Could you check a few things on this model? Use its own coordinates, in mm. Face numbers are marked on the shaded views. Coordinates: 2 decimals unless noted, no trailing zeros. Loops run counter-clockwise (first coordinate to the right, second up) from the corner with the lowest first, then second, coordinate; pieces in that order, holes last.
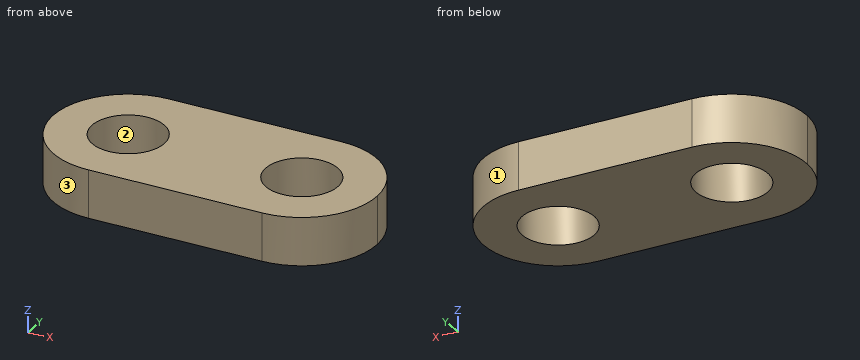
Autodesk Inventor part; units mm, degrees
ref_plane "YZ Plane" through (0, 0, 0) normal (1, 0, 0) x (0, 1, 0)
ref_plane "XZ Plane" through (0, 0, 0) normal (0, 1, 0) x (-1, 0, 0)
ref_plane "XY Plane" through (0, 0, 0) normal (0, 0, 1) x (1, 0, 0)
sketch "Sketch2" plane through (0, 0, 0) normal (0, 1, 0) x (-1, 0, 0)
  line L0 (0, -4.5) -> (-30.1, -4.5)
  line L1 (-30.1, -4.5) -> (-30.1, 0)
  line L2 (-30.1, 0) -> (0, 0)
  line L3 (0, 0) -> (0, -4.5)
  line L4 (-7, -4.5) -> (-7, 0) construction
  line L5 (-23.1, 0) -> (-23.1, -4.5) construction
  point P0 (-7, -2.25)
  point P1 (-23.1, -2.25)
  dimension "d7" = 16.1
  dimension "d8" = 4.5
  dimension "d9" = 7
  dimension "d11" = 7
extrude "Extrusion1" add sketch "Sketch2" along normal blind 14
sketch "Sketch3" plane through (0, 0, 0) normal (0, 0, 1) x (1, 0, 0)
  line L0 (30.1, 0) -> (30.1, 14)
  line L1 (0, 0) -> (0, 14)
  point P0 (7, 7)
  point P1 (23.1, 7)
  point P2 (30.1, 7)
  point P3 (7, 0)
  point P4 (23.1, 0)
hole "Hole1" at (7, 7, 0) at (23.1, 7, 0) direction (0, 0, -1) diameter 6.756 end through all
fillet "Fillet1" radius 7 4 edges at (0, 14, -2.25) (0, 0, -2.25) (30.1, 0, -2.25) (30.1, 14, -2.25)
properties part number "R3_3DPrint"
(1) For pin 1 (2 mm diameter, centred on y = 12.5, z = -1, fed in from +X); pin 2 (1.5 mm diameter, centred on y = 8, z = -0.5, fed in from +X), each with a flat end and sliding along its axis, tell me the tip position at first contact or that it passes through.
Answers:
pin 1: stops at x = 28.46
pin 2: stops at x = 30.1
(2) Imagine slicing it at C-C, the plane x = 6. Write out the boundary of the cut face in (y, z).
Answers:
outline: (0.07, -4.5) - (3.77, -4.5) - (3.77, 0) - (0.07, 0) - close; (10.23, -4.5) - (13.93, -4.5) - (13.93, 0) - (10.23, 0) - close
(3) Imagine slicing it at A-A, the plane z = -2.3. State how many separate pieces and enclosed holes the cut face has, and give its area (3 significant figures).
Answers:
separate pieces: 1
enclosed holes: 2
area: 308 mm2
(4) Imagine slicing it at B-B, the plane y = 4.25. Write out the boundary of the cut face in (x, z), and give its area (3 significant figures).
Answers:
outline: (0.56, -4.5) - (5.04, -4.5) - (5.04, 0) - (0.56, 0) - close; (8.96, -4.5) - (21.14, -4.5) - (21.14, 0) - (8.96, 0) - close; (25.06, -4.5) - (29.54, -4.5) - (29.54, 0) - (25.06, 0) - close
area: 95.1 mm2
(5) We'd pull the mould along X, two halves only. Please class the marked faces 1, 2 and 3: +X half, -X half, draft (parallel to the pull), parting line (faces both ways), or undercut.
Answers:
face 1: +X half
face 2: undercut
face 3: -X half
(6) Imagine slicing it at D-D, the plane y = 10. Write out the boundary of the cut face in (x, z).
Answers:
outline: (0.68, -4.5) - (5.45, -4.5) - (5.45, 0) - (0.68, 0) - close; (8.55, -4.5) - (21.55, -4.5) - (21.55, 0) - (8.55, 0) - close; (24.65, -4.5) - (29.42, -4.5) - (29.42, 0) - (24.65, 0) - close
(7) I need wall thicknesses on probe 1 along Y at (x, z) = (23.1, -1.55); probe 2 along X at (y, z) = (7.75, -2.9); probe 3 along X at (y, z) = (7, -0.3). Which ranges of each line are inside material? Lowest first, please.
Answers:
probe 1: y = 0 to 3.62, 10.38 to 14
probe 2: x = 0.04 to 3.71, 10.29 to 19.81, 26.39 to 30.06
probe 3: x = 0 to 3.62, 10.38 to 19.72, 26.48 to 30.1
